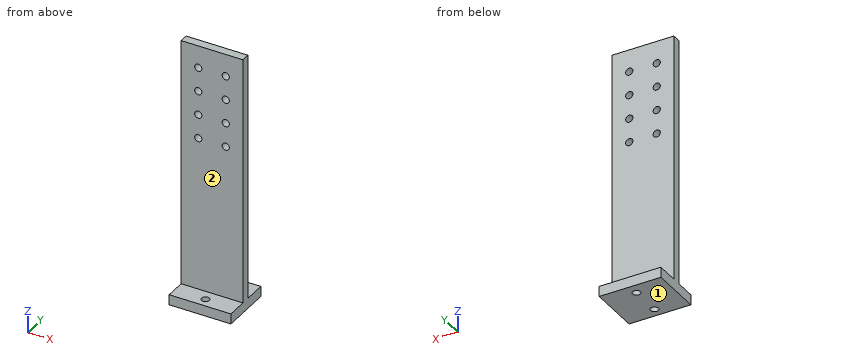
from build123d import *

# Parameters (mm, degrees)
BOX007_W          = 36
BOX007_H          = 5
BOX007_DEPTH      = 145
SKETCH001_R       = 2.1
POCKET001_DEPTH   = 5
CYLINDER003_R     = 2.25
CYLINDER003_DEPTH = 10
CYLINDER004_R     = 2.25
CYLINDER004_DEPTH = 10
BOX006_W          = 36
BOX006_H          = 30
BOX006_DEPTH      = 6


with BuildPart() as pocket001:
    # Box007 → Box007 (new body)
    with BuildSketch(Plane.XY):
        with Locations((18, 2.5)):
            Rectangle(BOX007_W, BOX007_H)
    extrude(amount=BOX007_DEPTH)

    # Sketch001 (on Face3 of Box007) → Pocket001 (cut)
    with BuildSketch(Plane.XZ):
        with Locations((10, 132)):
            Circle(SKETCH001_R)
        with Locations((26, 132)):
            Circle(SKETCH001_R)
        with Locations((10, 118)):
            Circle(SKETCH001_R)
        with Locations((26, 118)):
            Circle(SKETCH001_R)
        with Locations((10, 104)):
            Circle(SKETCH001_R)
        with Locations((26, 104)):
            Circle(SKETCH001_R)
        with Locations((10, 90)):
            Circle(SKETCH001_R)
        with Locations((26, 90)):
            Circle(SKETCH001_R)
    extrude(amount=-POCKET001_DEPTH, mode=Mode.SUBTRACT)


with BuildPart() as cilindro003:
    # Cylinder003 → Cylinder003 (new body)
    with BuildSketch(Plane(origin=(18, 11.5, -8), x_dir=(1, 0, 0), z_dir=(0, 0, 1))):
        Circle(CYLINDER003_R)
    extrude(amount=CYLINDER003_DEPTH)


with BuildPart() as cilindro004:
    # Cylinder004 → Cylinder004 (new body)
    with BuildSketch(Plane(origin=(18, -6.5, -8), x_dir=(1, 0, 0), z_dir=(0, 0, 1))):
        Circle(CYLINDER004_R)
    extrude(amount=CYLINDER004_DEPTH)


with BuildPart() as obj1:
    # Box006 → Box006 (new body)
    with BuildSketch(Plane(origin=(0, -12, -6), x_dir=(1, 0, 0), z_dir=(0, 0, 1))):
        with Locations((18, 15)):
            Rectangle(BOX006_W, BOX006_H)
    extrude(amount=BOX006_DEPTH)

    # Cut003001005: cut Cilindro004
    add(cilindro004.part, mode=Mode.SUBTRACT)

    # Cut003001006: cut Cilindro003
    add(cilindro003.part, mode=Mode.SUBTRACT)

    # Fusion001002018: union Pocket001
    add(pocket001.part)


solid = obj1.part
The model under review builds one solid part; all positions refer to its coordinate system, in mm. Face numbers are marked on the shaded views. Give positions to 0.01 mm unless a question says otherwise; leave off trailing zeros. Order: outer loops, then holes, each group sorted by start corner. A loop starts at its lowest first (then second) coordinate and runs counter-clockwise, first axis right, second up. Notation, with made-up numbers: (61, 2.25) -> (113, 2.25) arc R15 cw to (113, 7.25) -> close; hole circle Ø5 at (44, 84). An arc over 180 degrees is marked (long way). Write item = value, one per line. Start each with the question number.
(1) Take a section at D-D (x = 26). Write out the cut boundary in (y, z).
(2) Take a section at A-A (y = 11.5). Write out the cut boundary in (x, z).
(3) For pin 1 Ø2.5 at (x, z) = (26, 132) entering from +Y; pin 2 Ø3 at (x, z) = (17.5, 71) entering from +Y; pin 3 Ø6 at (x, z) = (29.5, 110) entering from -Y; pin 4 Ø5 at (x, y) = (18, -6.5) entering from +Z, all flat-tipped, find the tip position at first contact; note any pin that passes through.
(4) Take a section at C-C (z = 104). Write out the cut boundary in (x, y), plus the area to 3 significant figures.
(5) Take a section at B-B (x = 18). Write out the cut boundary in (y, z).
(6) Draft analysis for pull direction Z (two halves, no side actions). For the marked faces 1 and 2, state which applies: +Z half, -Z half, draft (parallel to the pull), parting line (faces both ways), or undercut.
(7) For L1, parallel to Y at x = 18, z = -2.15; L2, parallel to Z at x = 10, y = 3.25; L3, parallel to X at y = 1.6, z = 132, list the stretches that pass through material, from the lowest coordinate up. Write a range as from..to.
Returned:
q1.outline = (-12, -6) -> (18, -6) -> (18, 0) -> (5, 0) -> (5, 87.9) -> (0, 87.9) -> (0, 0) -> (-12, 0) -> close; (0, 92.1) -> (5, 92.1) -> (5, 101.9) -> (0, 101.9) -> close; (0, 106.1) -> (5, 106.1) -> (5, 115.9) -> (0, 115.9) -> close; (0, 120.1) -> (5, 120.1) -> (5, 129.9) -> (0, 129.9) -> close; (0, 134.1) -> (5, 134.1) -> (5, 145) -> (0, 145) -> close
q2.outline = (0, -6) -> (15.75, -6) -> (15.75, 0) -> (0, 0) -> close; (20.25, -6) -> (36, -6) -> (36, 0) -> (20.25, 0) -> close
q3.pin_1 = through
q3.pin_2 = 5
q3.pin_3 = 0
q3.pin_4 = 0
q4.outline = (0, 0) -> (7.9, 0) -> (7.9, 5) -> (0, 5) -> close; (12.1, 0) -> (23.9, 0) -> (23.9, 5) -> (12.1, 5) -> close; (28.1, 0) -> (36, 0) -> (36, 5) -> (28.1, 5) -> close
q4.area = 138 mm²
q5.outline = (-12, -6) -> (-8.75, -6) -> (-8.75, 0) -> (-12, 0) -> close; (-4.25, -6) -> (9.25, -6) -> (9.25, 0) -> (5, 0) -> (5, 145) -> (0, 145) -> (0, 0) -> (-4.25, 0) -> close; (13.75, -6) -> (18, -6) -> (18, 0) -> (13.75, 0) -> close
q6.face_1 = -Z half
q6.face_2 = draft
q7.L1 = -12..-8.75, -4.25..9.25, 13.75..18
q7.L2 = -6..87.9, 92.1..101.9, 106.1..115.9, 120.1..129.9, 134.1..145
q7.L3 = 0..7.9, 12.1..23.9, 28.1..36
